For this review, take the finished solid that the model builds, in its own axes (mm). Face numbers are marked on the shaded views. Give positions to 0.01 mm unless a question says otherwise; leave off trailing zeros. Order: outer loops, then holes, each group sorted by start corner. A loop starts at its lowest first (then second) coordinate and runs counter-clockwise, first axis right, second up. Notation, with made-up numbers: (42.25, 24) - (100.25, 24) arc R19 cw to (100.25, 54) - close; hole circle Ø7 at (40.5, 74.5). An arc over 180 degrees is marked (long way). Use a Markdown table: item, result. Add a question column.
1) We need section A-A on z = -292. Write out the cut boundary in (x, y), then the cut area to 3 significant figures.
2) Wall thickness on L1, parallel to Y at x = 0, z = 0.8; L2, parallel to Z at x = -33, y = -30; L3, parallel to X at y = 45, z = -487.5: over which ranges is each line inside the solid? List them lowest first.
3) Mouldability with a two-part tool opening along Y and no side actions: class the marked faces 1 and 2 as released by +Y, released by -Y, zero draft, split by the parting line, or undercut.
4) We need section B-B on x = -24. Write out the cut boundary in (y, z), then the cut area to 3 significant figures.
5) Clearance check with a flat-ended pin moving along its axis: P1, Ø11, axis at x = 0, y = 0, coming from the -Z side. State where the tip first meets the part, or that it passes through.
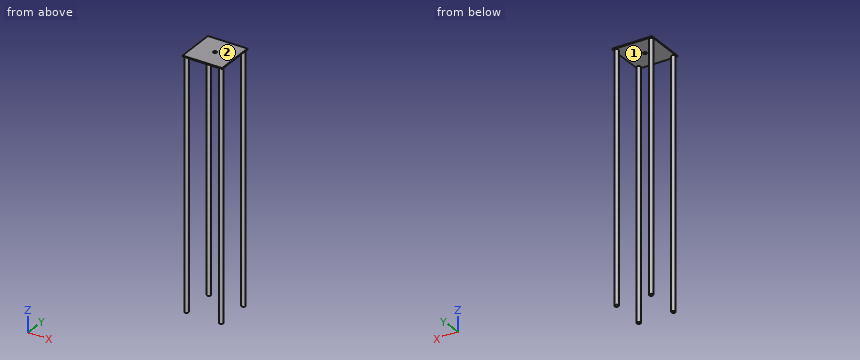
```python
from build123d import *

# Parameters (mm, degrees)
SKETCH1_W           = 101.6
SKETCH1_H           = 101.6
BOSS_EXTRUDE1_DEPTH = 2.54
SKETCH2_R           = 4.826
BOSS_EXTRUDE2_DEPTH = 635
SKETCH3_R           = 4.191
CUT_EXTRUDE1_DEPTH  = 635


with BuildPart() as part:
    # Sketch1 → Boss-Extrude1 (new body)
    with BuildSketch(Plane.XY):
        Rectangle(SKETCH1_W, SKETCH1_H)
    extrude(amount=BOSS_EXTRUDE1_DEPTH)

    # Sketch2 → Boss-Extrude2 (add)
    with BuildSketch(Plane(origin=(0, 0, 0), x_dir=(-1, 0, 0), z_dir=(0, 0, -1))):
        with Locations((-44.45, 44.45)):
            Circle(SKETCH2_R)
        with Locations((44.377290972, 44.45)):
            Circle(SKETCH2_R)
        with Locations((44.377290972, -44.45)):
            Circle(SKETCH2_R)
        with Locations((-44.45, -44.45)):
            Circle(SKETCH2_R)
    extrude(amount=BOSS_EXTRUDE2_DEPTH)

    # Sketch3 → Cut-Extrude1 (cut)
    with BuildSketch(Plane.XY.offset(2.54)):
        Circle(SKETCH3_R)
    extrude(amount=-CUT_EXTRUDE1_DEPTH, mode=Mode.SUBTRACT)


solid = part.part
```
Checked values:
| question | item | result |
|---|---|---|
| 1 | outline | circle Ø9.65 at (-44.38, -44.45); circle Ø9.65 at (-44.38, 44.45); circle Ø9.65 at (44.45, -44.45); circle Ø9.65 at (44.45, 44.45) |
| 1 | area | 293 mm² |
| 2 | L1 | -50.8 to -4.19, 4.19 to 50.8 |
| 2 | L2 | 0 to 2.54 |
| 2 | L3 | -49.17 to -39.58, 39.66 to 49.24 |
| 3 | face 1 | undercut |
| 3 | face 2 | zero draft |
| 4 | outline | (-50.8, 0) - (50.8, 0) - (50.8, 2.54) - (-50.8, 2.54) - close |
| 4 | area | 258 mm² |
| 5 | P1 | z = 0 |
